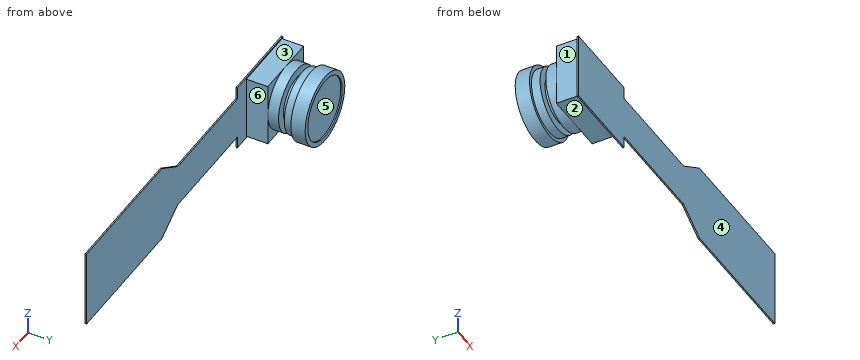
from build123d import *

# Parameters (mm, degrees)
SKETCH1_W           = 9
SKETCH1_H           = 9
BOSS_EXTRUDE1_DEPTH = 3
SKETCH2_R           = 4.5
BOSS_EXTRUDE2_DEPTH = 1.5
SKETCH3_R           = 3.25
BOSS_EXTRUDE3_DEPTH = 0.8
SKETCH4_R           = 4.5
BOSS_EXTRUDE4_DEPTH = 1.2
SKETCH6_R           = 5
BOSS_EXTRUDE5_DEPTH = 2
SKETCH7_R           = 4.344901587
CUT_EXTRUDE1_DEPTH  = 0.2
BOSS_EXTRUDE6_DEPTH = 0.2


with BuildPart() as part:
    # Sketch1 → Boss-Extrude1 (new body)
    with BuildSketch(Plane(origin=(0, 0, 0), x_dir=(1, 0, 0), z_dir=(0, 1, 0))):
        Rectangle(SKETCH1_W, SKETCH1_H)
    extrude(amount=BOSS_EXTRUDE1_DEPTH)

    # Sketch2 → Boss-Extrude2 (add)
    with BuildSketch(Plane(origin=(0, 3, 0), x_dir=(1, 0, 0), z_dir=(0, 1, 0))):
        with Locations(Location((0, 0, 0), (0, 0, 270))):
            Circle(SKETCH2_R)
    extrude(amount=BOSS_EXTRUDE2_DEPTH)

    # Sketch3 → Boss-Extrude3 (add)
    with BuildSketch(Plane(origin=(0, 4.5, 0), x_dir=(1, 0, 0), z_dir=(0, 1, 0))):
        with Locations(Location((0, 0, 0), (0, 0, 270))):
            Circle(SKETCH3_R)
    extrude(amount=BOSS_EXTRUDE3_DEPTH)

    # Sketch4 → Boss-Extrude4 (add)
    with BuildSketch(Plane(origin=(0, 5.3, 0), x_dir=(1, 0, 0), z_dir=(0, 1, 0))):
        with Locations(Location((0, 0, 0), (0, 0, 270))):
            Circle(SKETCH4_R)
    extrude(amount=BOSS_EXTRUDE4_DEPTH)

    # Sketch6 → Boss-Extrude5 (add)
    with BuildSketch(Plane(origin=(0, 6.5, 0), x_dir=(1, 0, 0), z_dir=(0, 1, 0))):
        with Locations(Location((0, 0, 0), (0, 0, 270))):
            Circle(SKETCH6_R)
    extrude(amount=BOSS_EXTRUDE5_DEPTH)

    # Sketch7 → Cut-Extrude1 (cut)
    with BuildSketch(Plane(origin=(0, 8.5, 0), x_dir=(1, 0, 0), z_dir=(0, 1, 0))):
        with Locations(Location((0, 0, 0), (0, 0, 270))):
            Circle(SKETCH7_R)
    extrude(amount=-CUT_EXTRUDE1_DEPTH, mode=Mode.SUBTRACT)

    # Sketch8 → Boss-Extrude6 (add)
    with BuildSketch(Plane.XZ):
        Polygon((6.8, 4.7), (6.8, 3), (21.8, 3), (25.8, 5.5), (44.8, 5.5), (44.8, -5.5), (25.8, -5.5), (21.8, -3), (6.8, -3), (6.8, -4.7), (-4.7, -4.7), (-4.7, 4.7), align=None)
    extrude(amount=BOSS_EXTRUDE6_DEPTH)


solid = part.part
Can you work these out from the model? Positions are in its coordinate system, mm. Face numbers are marked on the shaded views. A direction names the side the tool comes from. Round coordinates to 2 decimals unless told otherwise and drop trailing zeros. Loops run counter-clockwise (first coordinate to the right, second up) from the corner with the lowest first, then second, coordinate; pieces in that order, holes last. Notation, with made-up numbers: (-36, -36) - (-22, -36) arc R19 ccw to (-22, -19) - close; hole circle Ø6 at (-7.75, 16). An arc over 180 degrees is marked (long way). Use CSV: the item, a comma, the result in double quotes. Start each with the question number.
1) Please list where these lines run through material, in increasing order: probe 1 along X at (y, z) = (8.45, 0); probe 2 along Y at (x, z) = (1, -4); probe 3 along Y at (x, z) = (25, 2.75). Write a range as [from, to].
2) We'd pull the mould along X, two halves only. Please class the marked faces 4, 5 and 6: released by +X, released by -X, zero draft, split by the parting line, or undercut.
3) For the marked faces 1, 2 and 3, which set-ups out of +Z, -Z, +X, -X, +Y, -Y let a thin tool reach every point of the face, with its end or its side?
4) If we section it at D-D on z = -2.5: Write out the boundary of the cut face in (x, y).
5) For pin 1 Ø3.5 at (x, z) = (19, 2.5) entering from +Y; pin 2 Ø1.3 at (x, z) = (-3, 1.5) entering from +Y; pin 3 Ø1.5 at (y, z) = (6, -1) entering from +X; pin 4 Ø5 at (x, y) = (10, 3) entering from +Z, each with a flat end and sliding along its axis, tell me the tip position at first contact or that it passes through.
6) If we section it at C-C on y = 4: Write out the boundary of the cut face in (x, z), plus the area to 3 significant figures.
7) If we section it at B-B on x = 7.5: Write out the boundary of the cut face in (y, z).
Geometry results:
1,probe 1,"x = [-5, -4.34], [4.34, 5]"
1,probe 2,"y = [-0.2, 4.5], [5.3, 8.3]"
1,probe 3,"y = [-0.2, 0]"
2,face 4,"zero draft"
2,face 5,"undercut"
2,face 6,"released by +X"
3,face 1,"+Z, -Z, -X"
3,face 2,"-Z, +X, -X"
3,face 3,"+Z, +X, -X"
4,outline,"(-4.7, -0.2) - (44.8, -0.2) - (44.8, 0) - (4.5, 0) - (4.5, 3) - (3.74, 3) - (3.74, 4.5) - (2.08, 4.5) - (2.08, 5.3) - (3.74, 5.3) - (3.74, 6.5) - (4.33, 6.5) - (4.33, 8.5) - (3.55, 8.5) - (3.55, 8.3) - (-3.55, 8.3) - (-3.55, 8.5) - (-4.33, 8.5) - (-4.33, 6.5) - (-3.74, 6.5) - (-3.74, 5.3) - (-2.08, 5.3) - (-2.08, 4.5) - (-3.74, 4.5) - (-3.74, 3) - (-4.5, 3) - (-4.5, 0) - (-4.7, 0) - close"
5,pin 1,"stops at y = 0"
5,pin 2,"stops at y = 8.3"
5,pin 3,"stops at x = 4.98"
5,pin 4,"passes through"
6,outline,"circle Ø9 at (0, 0)"
6,area,"63.6 mm2"
7,outline,"(-0.2, -3) - (0, -3) - (0, 3) - (-0.2, 3) - close"
